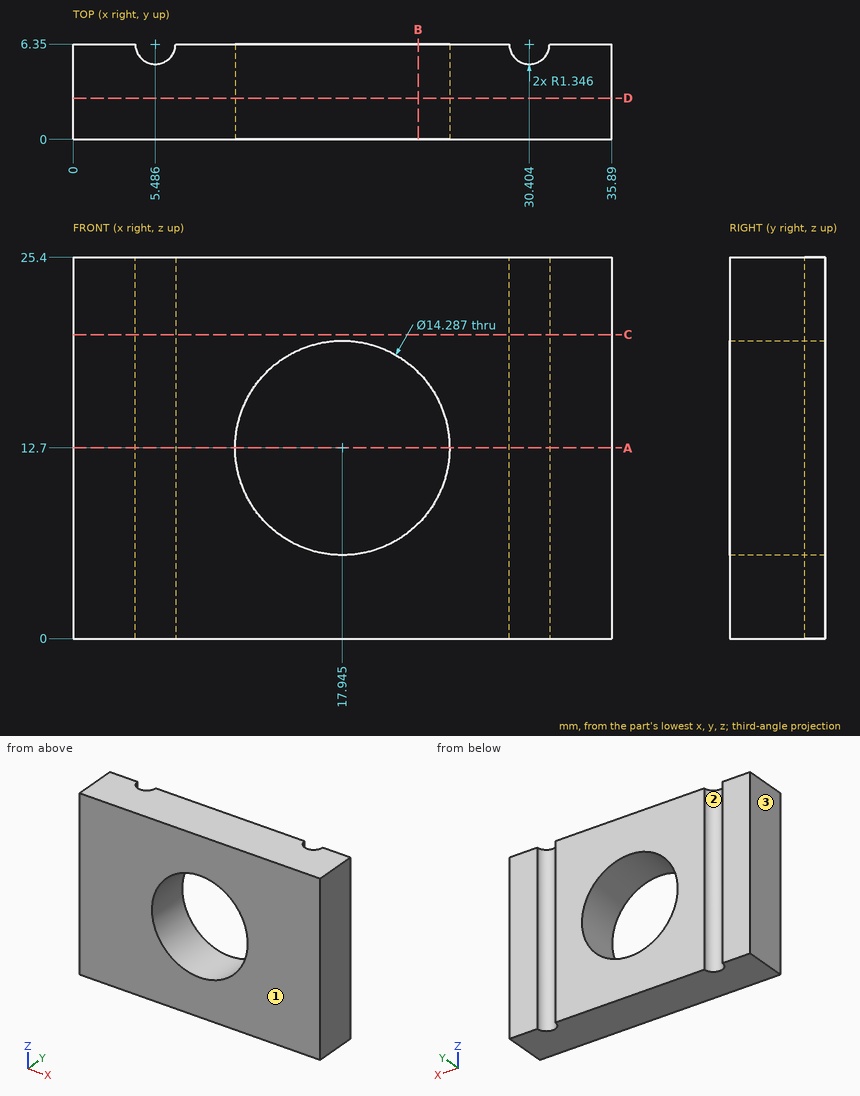
Geometry: see drawing. Coordinates: mm, zero at the bounding-box minimum. Coordinates: 2 decimals unless noted, no trailing zeros. Loops run counter-clockwise (first coordinate to the right, second up) from the corner with the lowest first, then second, coordinate; pieces in that order, holes last. Notation, with made-up numbers: (34.5, 19.25) -> (74.5, 19.25) arc R22 ccw to (74.5, 34.25) -> close; hole circle Ø5 at (-39.75, 50). An arc over 180 degrees is marked (long way). Write item = value, one per line. Start each with the question number.
Item 1: Cut plane A-A, the plane z = 12.7. Return loops of the section in (x, y).
Item 2: Cut plane B-B, the plane x = 23. Return loops of the section in (y, z).
Item 3: Cut plane C-C, the plane z = 20.25. Return loops of the section in (x, y), plus the area to 3 significant figures.
Item 4: Material intervals for line 1 (X direction, y = 4, z = 12.7); line 2 (X direction, y = 3, z = 7.75) (1 decimal); line 3 (Z direction, x = 19, y = 5.5) (1 decimal), sorted ascending.
Item 5: Cut plane D-D, the plane y = 2.75. Return loops of the section in (x, z) (1 decimal).
Item 6: Mould query, pull axis X, two halves, no side actions, for the marked faces 1, 2 and 3. Classes: pulls with the +X half, pulls with the -X half, needs draft (parallel to the pull), parting line crosses it, or undercut.
Ans:
q1.outline = (0, 0) -> (10.8, 0) -> (10.8, 6.35) -> (6.83, 6.35) arc R1.35 cw to (4.14, 6.35) -> (0, 6.35) -> close; (25.09, 0) -> (35.89, 0) -> (35.89, 6.35) -> (31.75, 6.35) arc R1.35 cw to (29.06, 6.35) -> (25.09, 6.35) -> close
q2.outline = (0, 0) -> (6.35, 0) -> (6.35, 7.65) -> (0, 7.65) -> close; (0, 17.75) -> (6.35, 17.75) -> (6.35, 25.4) -> (0, 25.4) -> close
q3.outline = (0, 0) -> (35.89, 0) -> (35.89, 6.35) -> (31.75, 6.35) arc R1.35 cw to (29.06, 6.35) -> (6.83, 6.35) arc R1.35 cw to (4.14, 6.35) -> (0, 6.35) -> close
q3.area = 222 mm²
q4.line_1 = 0 to 10.8, 25.09 to 35.89
q4.line_2 = 0 to 12.8, 23.1 to 35.9
q4.line_3 = 0 to 5.6, 19.8 to 25.4
q5.outline = (0, 0) -> (35.9, 0) -> (35.9, 25.4) -> (0, 25.4) -> close; hole circle Ø14.3 at (17.9, 12.7)
q6.face_1 = needs draft
q6.face_2 = undercut
q6.face_3 = pulls with the -X half
